Source: three-view drawing plus pictorial views. Frame: mm from the lowest corner of the part. A direction names the side the tool comes from. Give positions to 0.01 mm unless a question says otherwise; leave off trailing zeros. Order: outer loops, then holes, each group sorted by start corner. A loop starts at its lowest first (then second) coordinate and runs counter-clockwise, first axis right, second up. Notation, with made-up numbers: (43, 23) - (60, 23) arc R29 ccw to (60, 48) - close; hole circle Ø3 at (15.25, 41). An arc over 180 degrees is marked (long way). Answer in a Markdown table with one row per item. Add a question column.
1. Access query for the marked faces 1, 2 and 3. Directions: +Z, -Z, +X, -X, +Y, -Y. A direction counts if a zero-diameter tool reaches every point of the face in a straight line with its end or side. Return the directions, or none.
2. Section query A-A on x = 3.25. Return loops of the section in (y, z), and give its area (4 significant figures).
3. Section query C-C on y = 15.5. Return loops of the section in (x, z).
4. Contact query for flat-ended pins moving along their axis: pin 1 (2 mm diameter, centred on y = 20, z = 4.5, fed in from +X); pin 2 (0.5 mm diameter, centred on x = 3.5, y = 39, fed in from +Z); pin 3 (0.5 mm diameter, centred on y = 4, z = 5, fed in from +X). Output: stop coordinate, or through.
5. Ray query, line 1 (Y direction, x = 5, z = 2.75); line 2 (Z direction, x = 3, y = 13); line 3 (X direction, y = 17, z = 4.5). Return the intervals inside material, ascending. Write a range as [from, to].
6. Section query B-B on z = 3.25. Return loops of the section in (x, y).
7. Section query D-D on y = 35.5. Return loops of the section in (x, z), and give its area (3 significant figures).
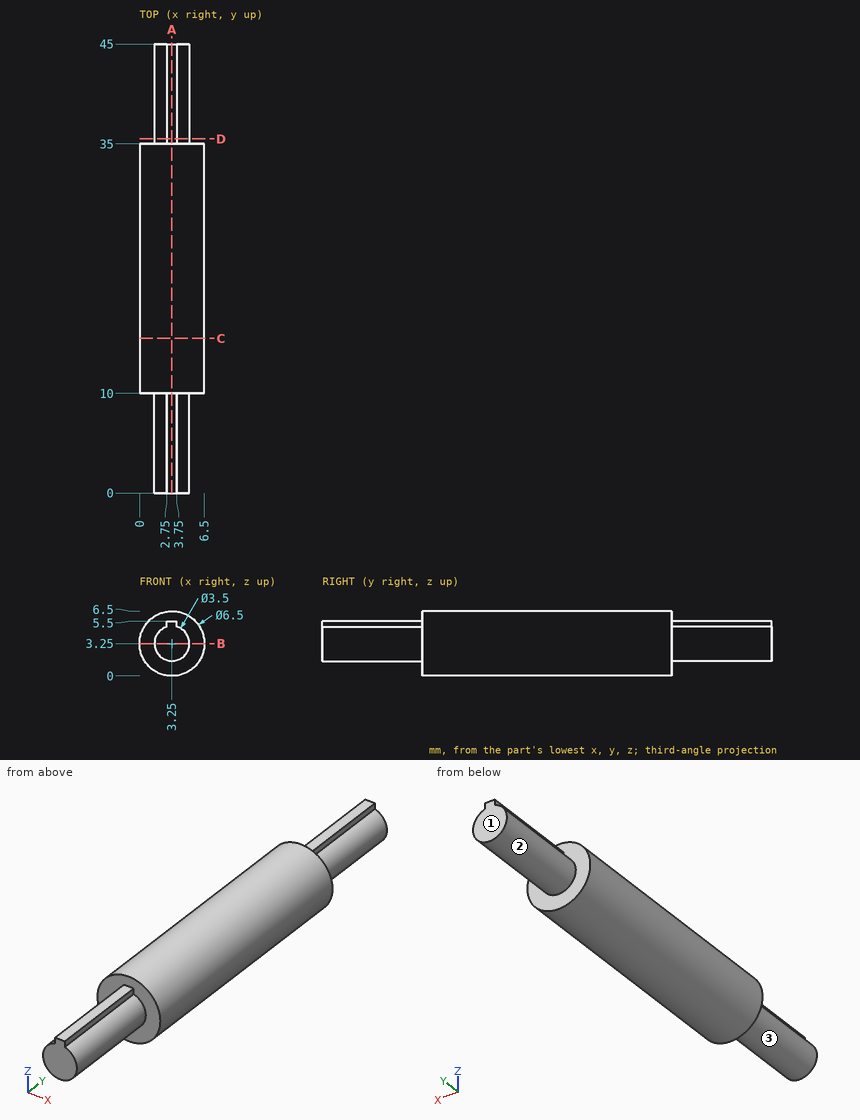
Answer:
| question | item | result |
|---|---|---|
| 1 | face 1 | +Z, -Z, +X, -X, +Y |
| 1 | face 2 | +Y |
| 1 | face 3 | -Y |
| 2 | outline | (0, 1.5) - (10, 1.5) - (10, 0) - (35, 0) - (35, 1.5) - (45, 1.5) - (45, 5.5) - (35, 5.5) - (35, 6.5) - (10, 6.5) - (10, 5.5) - (0, 5.5) - close |
| 2 | area | 242.5 mm² |
| 3 | outline | circle Ø6.5 at (3.25, 3.25) |
| 4 | pin 1 | stops at x = 6.49 |
| 4 | pin 2 | stops at z = 5.5 |
| 4 | pin 3 | stops at x = 4.15 |
| 5 | line 1 | y = [10, 35] |
| 5 | line 2 | z = [0.01, 6.49] |
| 5 | line 3 | x = [0.25, 6.25] |
| 6 | outline | (0, 10) - (1.5, 10) - (1.5, 0) - (5, 0) - (5, 10) - (6.5, 10) - (6.5, 35) - (5, 35) - (5, 45) - (1.5, 45) - (1.5, 35) - (0, 35) - close |
| 7 | outline | (2.75, 4.93) arc R1.75 ccw (long way) to (3.75, 4.93) - (3.75, 5.5) - (2.75, 5.5) - close |
| 7 | area | 10.1 mm² |
